For this review, take the finished solid that the model builds, in its own axes (mm). Face numbers are marked on the shaded views. A direction names the side the tool comes from. Round coordinates to 2 decimals unless told otherwise and drop trailing zeros. Write each loop counter-clockwise with the first axis right and the second up, starting at its lowest first coordinate (ties: lowest second). Pieces come first, ordered by that corner, then holes. Notation, with made-up numbers: (16.5, 58) -> (42.5, 58) arc R12 cw to (42.5, 75) -> close; hole circle Ø2 at (22, -4.5). An arc over 180 degrees is marked (long way). Write item = value, one per line. Start each with the question number.
```python
from build123d import *

# Parameters (mm, degrees)
FILLET1_R           = 0.1
FILLET2_R           = 0.15
HEX_2_DEPTH         = 1.3
SKETCH4_R           = 1.55
BOSS_EXTRUDE1_DEPTH = 15


with BuildPart() as part:
    # BodySke → Base-Revolve (revolve)
    with BuildSketch(Plane.XY):
        Polygon((0, 0), (0, 2.75), (3, 2.75), (3, 1.5), (22.7195, 1.5), (23, 1.2195), (23, 0), align=None)
    revolve(axis=Axis((-31.75, 0, 0), (1, 0, 0)))

    # Fillet1
    fillet1_edges = [part.edges().sort_by_distance(p)[0] for p in [
        (3, -1.5, 0),
    ]]
    fillet(fillet1_edges, radius=FILLET1_R)

    # Fillet2
    fillet2_edges = [part.edges().sort_by_distance(p)[0] for p in [
        (0, -2.75, 0),
    ]]
    fillet(fillet2_edges, radius=FILLET2_R)

    # Sketch2 → Hex-PreBroach (revolve, cut)
    with BuildSketch(Plane.XY):
        Polygon((0, 1.28), (1.3, 1.28), (2.039008345, 0), (0, 0), align=None)
    revolve(axis=Axis((0, 0, 0), (1, 0, 0)), mode=Mode.SUBTRACT)

    # Sketch3 → Hex 2 (cut)
    with BuildSketch(Plane(origin=(0, 0, 0), x_dir=(0, 0.5, 0.866025404), z_dir=(-1, 0, 0))):
        Polygon((0.739008345, 1.28), (-0.739008345, 1.28), (-1.478016689, 0), (-0.739008345, -1.28), (0.739008345, -1.28), (1.478016689, 0), align=None)
    extrude(amount=-HEX_2_DEPTH, mode=Mode.SUBTRACT)

    # Sketch4 → Boss-Extrude1 (add)
    with BuildSketch(Plane(origin=(3, 0, 0), x_dir=(0, 0, -1), z_dir=(1, 0, 0))):
        Circle(SKETCH4_R)
    extrude(amount=BOSS_EXTRUDE1_DEPTH)


solid = part.part
```
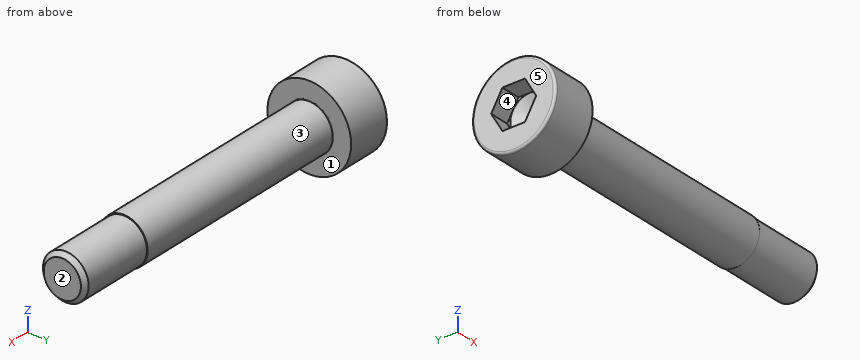
1. Draft analysis for pull direction Y (two halves, no side actions). For the marked faces 3, 4 and 5, state which applies: +Y half, -Y half, draft (parallel to the pull), parting line (faces both ways), or undercut.
2. Consider section A-A, the plane x = 14.25. Give the boundary of the cut face in (y, z).
3. Machinability: for the marked faces 1 and 2, which of the approach directions +Z, -Z, +X, -X, +Y, -Y give a long, thin tool a straight path to every point of the face, cutting with its end or side? Answer none if there is none.
4. Clearance check with flat-ended pins moving along their axes: pin 1 Ø1.5 at (x, y) = (17.5, 1.5) entering from +Z; pin 2 Ø2 at (x, y) = (13.5, 1) entering from +Z; pin 3 Ø1 at (x, y) = (5, -0.5) entering from -Z. State where each tip first meets the part, or that it passes through.
5. Wall thickness on L1, parallel to X at y = 1.6, z = 0.4; L2, parallel to Z at x = 16.5, y = 0.05; L3, parallel to Z at x = 7.75, y = -0.6: over which ranges is each line inside the solid? List them lowest first. Write a range as from..to.
Outcome:
q1.face_3 = parting line
q1.face_4 = undercut
q1.face_5 = draft
q2.outline = circle Ø3.1 at (0, 0)
q3.face_1 = +X
q3.face_2 = +Z, -Z, +X, +Y, -Y
q4.pin_1 = 1.36
q4.pin_2 = 1.55
q4.pin_3 = -1.55
q5.L1 = 0..3
q5.L2 = -1.55..1.55
q5.L3 = -1.43..1.43
